Autodesk Inventor part; units mm, degrees
ref_plane "YZ Plane" through (0, 0, 0) normal (1, 0, 0) x (0, 1, 0)
ref_plane "XZ Plane" through (0, 0, 0) normal (0, 1, 0) x (-1, 0, 0)
ref_plane "XY Plane" through (0, 0, 0) normal (0, 0, 1) x (1, 0, 0)
sketch "Sketch1" plane through (0, 0, 0) normal (0, 0, 1) x (1, 0, 0)
  arc A0 (107.7631, -107.7631) -> (-107.7631, 107.7631) centre (0, 0) ccw
  line L0 (152.4, 0) -> (127, 0)
  line L1 (127, -1.66) -> (127, 1.66)
  line L2 (127, 1.66) -> (50.7729, 1.66)
  line L3 (50.7729, -1.66) -> (127, -1.66)
  line L4 (-64.9376, 109.1552) -> (-26.824, 43.1406)
  line L5 (-23.9488, 44.8006) -> (-62.0624, 110.8152)
  line L6 (-1.66, 127) -> (-1.66, 50.7729)
  line L7 (1.66, 50.7729) -> (1.66, 127)
  line L8 (1.66, 127) -> (-1.66, 127)
  line L9 (-62.0624, 110.8152) -> (-64.9376, 109.1552)
  line L10 (35.921, 35.921) -> (107.7631, 107.7631)
  line L11 (0, 0) -> (152.4, 0) construction
  line L12 (0, 0) -> (152.4, 0) construction
  line L13 (107.7631, -107.7631) -> (35.921, -35.921)
  line L14 (-35.921, 35.921) -> (-107.7631, 107.7631)
  arc A1 (-26.824, 43.1406) -> (-35.921, 35.921) centre (0, 0) ccw
  arc A2 (35.921, -35.921) -> (1.66, 50.7729) centre (0, 0) ccw
  arc A3 (-1.66, 50.7729) -> (-23.9488, 44.8006) centre (0, 0) ccw
  line L15 (35.921, 35.921) -> (53.5987, 53.5987)
  line L16 (107.7631, 107.7631) -> (90.0854, 90.0854)
  circle A4 centre (53.5987, 53.5987) radius 15
  line L17 (53.5987, 53.5987) -> (58.902, 48.2954)
  line L18 (53.5987, 53.5987) -> (48.2954, 58.902)
  circle A5 centre (48.2954, 58.902) radius 2.5
  circle A6 centre (58.902, 48.2954) radius 2.5
  circle A7 centre (90.0854, 90.0854) radius 15
  line L19 (90.0854, 90.0854) -> (95.3887, 84.7821)
  line L20 (90.0854, 90.0854) -> (84.7821, 95.3887)
  circle A8 centre (84.7821, 95.3887) radius 2.5
  circle A9 centre (95.3887, 84.7821) radius 2.5
  line L21 (-90.0854, 90.0854) -> (-84.7821, 95.3887)
  circle A10 centre (-84.7821, 95.3887) radius 2.5
  circle A11 centre (-90.0854, 90.0854) radius 15
  line L22 (-90.0854, 90.0854) -> (-95.3887, 84.7821)
  circle A12 centre (-95.3887, 84.7821) radius 2.5
  circle A13 centre (-58.902, 48.2954) radius 2.5
  circle A14 centre (-53.5987, 53.5987) radius 15
  line L23 (-53.5987, 53.5987) -> (-58.902, 48.2954)
  circle A15 centre (-48.2954, 58.902) radius 2.5
  line L24 (-53.5987, 53.5987) -> (-48.2954, 58.902)
  line L25 (90.0854, -90.0854) -> (84.7821, -95.3887)
  circle A16 centre (84.7821, -95.3887) radius 2.5
  circle A17 centre (90.0854, -90.0854) radius 15
  line L26 (90.0854, -90.0854) -> (95.3887, -84.7821)
  circle A18 centre (95.3887, -84.7821) radius 2.5
  circle A19 centre (58.902, -48.2954) radius 2.5
  circle A20 centre (53.5987, -53.5987) radius 15
  line L27 (53.5987, -53.5987) -> (58.902, -48.2954)
  circle A21 centre (48.2954, -58.902) radius 2.5
  line L28 (53.5987, -53.5987) -> (48.2954, -58.902)
  point P0 (50.8, 0)
  dimension "d2" = 25.4
  dimension "d3" = 3.32
  dimension "d10" = 45
  dimension "d12" = 25
  dimension "d13" = 25
  dimension "d14" = 30
  dimension "d15" = 7.5
  dimension "d16" = 7.5
  dimension "d17" = 5
  dimension "d18" = 5
  dimension "d19" = 30
  dimension "d20" = 7.5
  dimension "d21" = 7.5
  dimension "d22" = 5
  dimension "d23" = 5
extrude "Extrusion5" add sketch "Sketch1" along normal mid plane 4 contours L13 A17 A20 A2 L3 L1 L0 A0 | L0 L1 L2 A2 L10 A4 A7 A0 | L13 A17 | A7 L10 | L13 A20 | A4 L10 picked at (87.4853, -84.823) picked at (87.4853, 84.823) picked at (50.9986, -48.3363) picked at (50.9986, 48.3363)
fillet "Fillet2" radius 2 6 edges at (46.6091, -20.2046, -2) (46.6091, -20.2046, 2) (46.6091, 20.2046, -2) (46.6091, 20.2046, 2) (152.4, 0, -2) (152.4, 0, 2)
properties part number "fin_alignment_rig_part2"
Verification items for the finished model (mm, model axes). A direction names the side the tool comes from. Coordinates: 2 decimals unless noted, no trailing zeros. Loops run counter-clockwise (first coordinate to the right, second up) from the corner with the lowest first, then second, coordinate; pieces in that order, holes last. Notation, with made-up numbers: (64, 85) -> (84, 85) arc R22 ccw to (84, 98) -> close; hole circle Ø6 at (41, -36). An arc over 180 degrees is marked (long way). Answer as a JSON object with one key per item and string values. Group by question number.
Item 1: Tool access check on faces 4 (the flat face through (71, 71, 0)), 5 (the flat face through (89, 1.66, 0)). Record the directions out of +Z, -Z, +X, -X, +Y, -Y that give a thin tool (end or side, any length) a straight path to the whole face; none if there is none.
Item 2: Scan lines: probe 1 along X at (y, z) = (85, 0.9); probe 2 along Y at (x, z) = (70.5, -1.05); probe 3 along Y at (x, z) = (83, 1.4). Record each from-to range of solid material in increasing order.
Item 3: Mould release check, pull along X, two halves, no side actions. Record for faces 1 (the flat face through (106, -22, -2)), 2 (the flat face through (72, -72, 0)), 3 (the cylindrical face through (61.287, 47.544, -0.028)): +X half, -X half, draft (parallel to the pull), parting line (faces both ways), or undercut.
Item 4: Sectioned sample at C-C on z = -1.35. Record the boundary of the cut face in (x, y), plus the area to 3 significant figures.
Item 5: Sectioned sample at A-A on x = 82.5. Record the boundary of the cut face in (y, z), plus the area to 3 significant figures.
Item 6: Depth check by flat-ended pin: pin 1 (6.5 mm diameter, centred on x = 95.39, y = -84.78, fed in from -Z); pin 2 (2 mm diameter, centred on x = 83, z = 0, fed in from -Y); pin 3 (1 mm diameter, centred on y = 0.5, z = 0.5, fed in from -X); pin 4 (2 mm diameter, centred on x = 93, z = 1, fed in from +Y). Enter the tip coordinate at first touch or a pass-through.
Item 7: Sectioned sample at B-B on x = 68. Record the boundary of the cut face in (y, z).
Evaluation:
{
 "1": {"face 4": "+Z, -Z, -X, +Y", "face 5": "+Z, -Z, -X"},
 "2": {"probe 1": "x = 85 to 92.9, 97.88 to 126.24", "probe 2": "y = -70.5 to -1.66, 1.66 to 70.5", "probe 3": "y = -83 to -1.66, 1.66 to 83"},
 "3": {"face 1": "draft", "face 2": "-X half", "face 3": "undercut"},
 "4": {"outline": "(36.29, -36.29) -> (107.39, -107.39) arc R151.88 ccw to (107.39, 107.39) -> (36.29, 36.29) arc R51.32 cw to (51.3, 1.66) -> (127, 1.66) -> (127, -1.66) -> (51.3, -1.66) arc R51.32 cw to start; hole circle Ø5 at (58.9, -48.3); hole circle Ø5 at (58.9, 48.3); hole circle Ø5 at (95.39, -84.78); hole circle Ø5 at (95.39, 84.78)", "area": "15,700 mm²"},
 "5": {"outline": "(-82.5, -2) -> (-1.66, -2) -> (-1.66, 2) -> (-82.5, 2) -> close; (1.66, -2) -> (82.5, -2) -> (82.5, 2) -> (1.66, 2) -> close", "area": "647 mm²"},
 "6": {"pin 1": "stops at z = -2", "pin 2": "stops at y = -84", "pin 3": "stops at x = 127", "pin 4": "stops at y = 94"},
 "7": {"outline": "(-68, -2) -> (-1.66, -2) -> (-1.66, 2) -> (-68, 2) -> close; (1.66, -2) -> (68, -2) -> (68, 2) -> (1.66, 2) -> close"}
}
